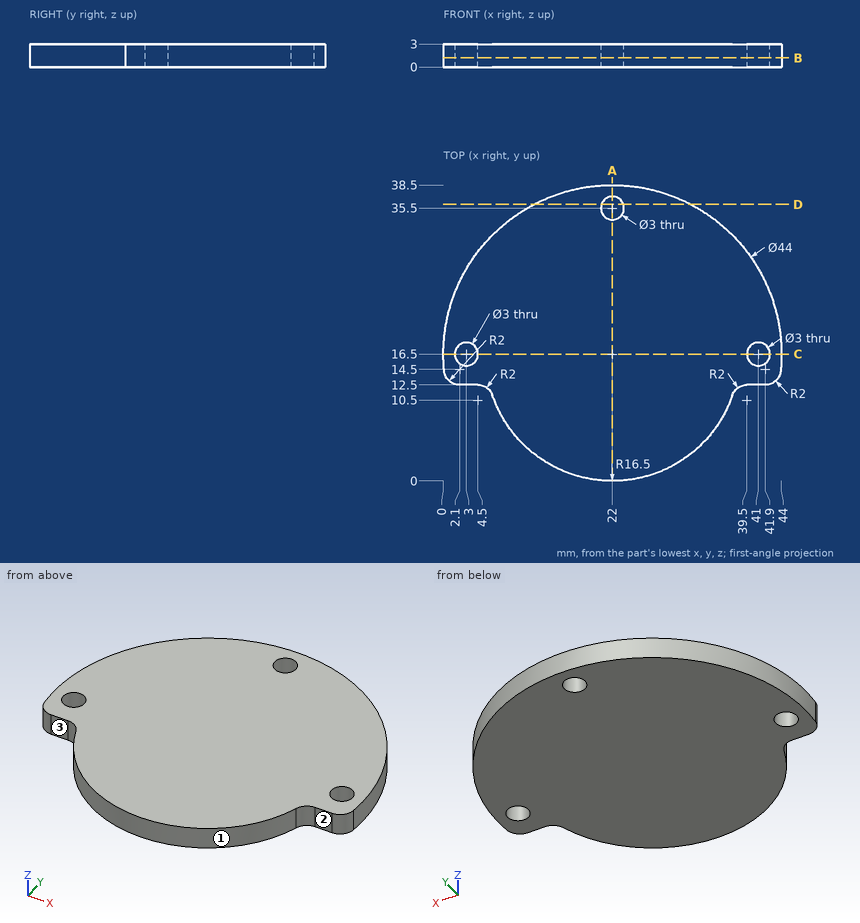
Check sheet for the drawn part. Datum: minimum x, y, z corner. Units: mm. A direction names the side the tool comes from. Coordinates: 2 decimals unless noted, no trailing zeros. Order: outer loops, then holes, each group sorted by start corner. A loop starts at its lowest first (then second) coordinate and runs counter-clockwise, first axis right, second up. Notation, with made-up numbers: (22.5, 58.5) -> (36.5, 58.5) arc R26 cw to (36.5, 94.5) -> close; hole circle Ø5 at (36, -8). An arc over 180 degrees is marked (long way). Write each question's results on one line, items separated by ' | '. Start each with the question number.
1) Material ranges on line 1 along Y through (x, z) = (3, 1.2); line 2 along X through (y, z) = (16, 2.9) (1 decimal); line 3 along X through (y, z) = (36, 1.2) (1 decimal), recorded low to high.
2) Section check A-A (x = 22). Enter the section's corners in (y, z), and give its area (4 significant figures).
3) Section check C-C (y = 16.5). Enter the section's corners in (x, z), and give its area (3 significant figures).
4) Depth check by flat-ended pin: pin 1 (2.5 mm diameter, centred on x = 41, y = 16.5, fed in from -Z); pin 2 (5 mm diameter, centred on x = 21.5, y = 7.5, fed in from -Z). Enter the tip coordinate at first touch or a pass-through.
5) Set-up check for the marked faces 1, 2 and 3: record each of +Z, -Z, +X, -X, +Y, -Y from which the full face is reachable in a straight line by a thin tool's end or side.
6) Section check B-B (z = 1.2). Enter the section's corners in (x, y).
7) Section check D-D (y = 36). Enter the section's corners in (x, z).
Checked values:
1) line 1: 12.5 to 15, 18 to 27.59 | line 2: 0 to 1.6, 4.4 to 39.6, 42.4 to 44 | line 3: 11.8 to 20.6, 23.4 to 32.2
2) outline: (0, 0) -> (34, 0) -> (34, 3) -> (0, 3) -> close; (37, 0) -> (38.5, 0) -> (38.5, 3) -> (37, 3) -> close | area: 106.5 mm²
3) outline: (0, 0) -> (1.5, 0) -> (1.5, 3) -> (0, 3) -> close; (4.5, 0) -> (39.5, 0) -> (39.5, 3) -> (4.5, 3) -> close; (42.5, 0) -> (44, 0) -> (44, 3) -> (42.5, 3) -> close | area: 114 mm²
4) pin 1: through | pin 2: z = 0
5) face 1: +Z, -Z, -Y | face 2: +Z, -Z, +X, -Y | face 3: +Z, -Z, -X, -Y
6) outline: (0.11, 14.3) arc R2 ccw to (2.1, 12.5) -> (4.5, 12.5) arc R2 cw to (6.39, 11.15) arc R16.5 ccw to (37.61, 11.15) arc R2 cw to (39.5, 12.5) -> (41.9, 12.5) arc R2 ccw to (43.89, 14.3) arc R22 ccw (long way) to start; hole circle Ø3 at (3, 16.5); hole circle Ø3 at (22, 35.5); hole circle Ø3 at (41, 16.5)
7) outline: (11.81, 0) -> (20.59, 0) -> (20.59, 3) -> (11.81, 3) -> close; (23.41, 0) -> (32.19, 0) -> (32.19, 3) -> (23.41, 3) -> close
